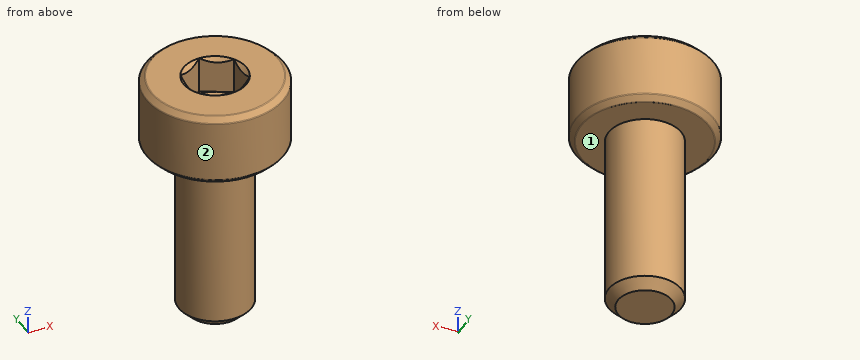
from build123d import *

# Parameters (mm, degrees)
CUT_EXTRUDE1_DEPTH = 1


with BuildPart() as part:
    # Sketch3 → Revolve1 (revolve)
    with BuildSketch(Plane(origin=(0, 0, 0), x_dir=(0, 0, -1), z_dir=(1, 0, 0)), mode=Mode.PRIVATE) as revolve1_sk:
        with BuildLine():
            Line((-3.5, 1.732259885), (-3.5, 0.75))
            Line((-3.5, 0.75), (-2.5, 0.75))
            Line((-2.5, 0.75), (-2.5, 0))
            Line((-2.5, 0), (3.5, 0))
            Line((3.5, 0), (3.5, 0.740192379))
            Line((3.5, 0.740192379), (3.240192379, 1))
            Line((3.240192379, 1), (-1.5, 1))
            Line((-1.5, 1), (-1.5, 1.732259885))
            ThreePointArc((-1.5, 1.732259885), (-1.502892578, 1.746801855), (-1.511129942, 1.759129942))
            Line((-1.511129942, 1.759129942), (-1.640870058, 1.888870058))
            ThreePointArc((-1.640870058, 1.888870058), (-1.653198145, 1.897107422), (-1.667740115, 1.9))
            Line((-1.667740115, 1.9), (-3.332259885, 1.9))
            ThreePointArc((-3.332259885, 1.9), (-3.346801855, 1.897107422), (-3.359129942, 1.888870058))
            Line((-3.359129942, 1.888870058), (-3.488870058, 1.759129942))
            ThreePointArc((-3.488870058, 1.759129942), (-3.497107422, 1.746801855), (-3.5, 1.732259885))
        make_face()
    revolve(revolve1_sk.sketch.rotate(Axis((0, 0, 3.5), (0, 0, -1)), 180), axis=Axis((0, 0, 3.5), (0, 0, -1)))

    # Sketch4 → Cut-Extrude1 (cut)
    with BuildSketch(Plane.XY.offset(3.5)):
        Polygon((0, 0.866025404), (-0.75, 0.433012702), (-0.75, -0.433012702), (0, -0.866025404), (0.75, -0.433012702), (0.75, 0.433012702), align=None)
    extrude(amount=-CUT_EXTRUDE1_DEPTH, mode=Mode.SUBTRACT)

    # Cut-Extrude2 cone 1 section (through the dimple's axis) → Cut-Extrude2 (revolve, cut)
    with BuildSketch(Plane(origin=(0, 0, 3.5), x_dir=(0, -1, 0), z_dir=(1, 0, 0))):
        Polygon((0, 0), (0.866025404, 0), (0, 0.866025404), align=None)
    revolve(axis=Axis((0, 0, 3.5), (0, 0, -1)), mode=Mode.SUBTRACT)

    # Cut-Extrude3 cone 1 section (through the dimple's axis) → Cut-Extrude3 (revolve, cut)
    with BuildSketch(Plane(origin=(0, 0, 2.5), x_dir=(0, -1, 0), z_dir=(1, 0, 0))):
        Polygon((0, 0), (0.75, 0), (0, 0.433012702), align=None)
    revolve(axis=Axis((0, 0, 2.5), (0, 0, -1)), mode=Mode.SUBTRACT)


solid = part.part
Could you check a few things on this model? Use its own coordinates, in mm. Face numbers are marked on the shaded views. A direction names the side the tool comes from. Coordinates: 2 decimals unless noted, no trailing zeros. Loops run counter-clockwise (first coordinate to the right, second up) from the corner with the lowest first, then second, coordinate; pieces in that order, holes last.
1. For the marked faces 1 and 2, which set-ups out of +Z, -Z, +X, -X, +Y, -Y let a thin tool reach every point of the face, with its end or its side?
2. Imagine slicing it at B-B (z = -0.25). Please give me the cut outline in (x, y), and give its area (3 significant figures).
3. Imagine slicing it at A-A (z = 2.75). Please give me the cut outline in (x, y).
4. For P1, Ø2, axis at x = 1, y = 0.5, coming from the -Z side; P2, Ø1.5, axis at y = -1, z = -1, coming from the +X side; P3, Ø1.5, axis at x = 1.5, z = 0.5, coming from the -Y side, each with a flat end and sliding along its axis, tell me the tip position at first contact or that it passes through.
5. I need wall thicknesses on L1, parallel to Z at x = 0.75, y = 1.15; L2, parallel to Y at x = 0.9, z = -1.75; L3, parallel to Y at x = -0.45, z = 3. Which ranges of each line are inside material? Lowest first, please.
Computed values:
1. face 1: -Z
1. face 2: +Z, -Z
2. outline: circle Ø2 at (0, 0)
2. area: 3.14 mm2
3. outline: circle Ø3.8 at (0, 0); hole (-0.75, -0.43) - (0, -0.87) - (0.75, -0.43) - (0.75, 0.43) - (0, 0.87) - (-0.75, 0.43) - close
4. P1: stops at z = -3.5
4. P2: stops at x = 0.97
4. P3: stops at y = -0.66
5. L1: z = 1.5 to 3.5
5. L2: y = -0.44 to 0.44
5. L3: y = -1.85 to -0.61, 0.61 to 1.85
